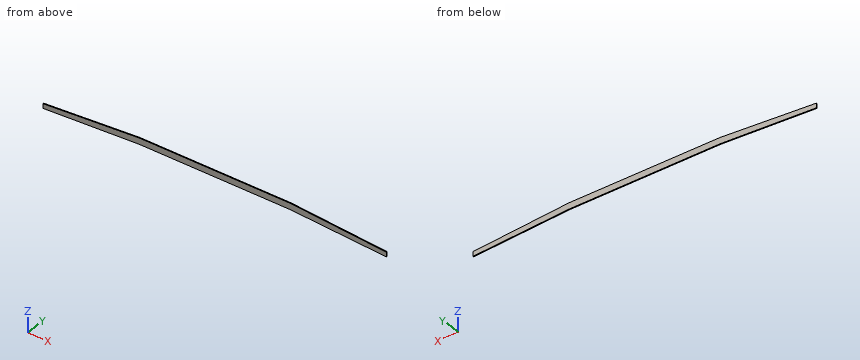
from build123d import *

# Parameters (mm, degrees)
BOSS_EXTRUDE1_DEPTH = 4.3


with BuildPart() as part:
    # Sketch1 → Boss-Extrude1 (new body)
    with BuildSketch(Plane(origin=(0, 0, 0), x_dir=(1, 0, 0), z_dir=(0, 1, 0))):
        Polygon((335.3, -13.5), (762, 17.8), (762, 37.8), (335.3, 13.5), (0, 13.5), (0, -13.5), align=None)
    boss_extrude1 = extrude(amount=BOSS_EXTRUDE1_DEPTH)

    # Mirror1: Boss-Extrude1 across plane
    add(boss_extrude1.mirror(Plane(origin=(0, 4.3, -13.5), x_dir=(0, 0, 1), z_dir=(1, 0, 0))))


solid = part.part
Input: part model. Units: mm. Frame: model coordinates. Round coordinates to 2 decimals unless told otherwise and drop trailing zeros. Write each loop counter-clockwise with the first axis right and the second up, starting at its lowest first coordinate (ties: lowest second). Pieces come first, ordered by that corner, then holes.
1) Cut plane B-B (x = -124). Return the cut outline in (y, z).
2) Contact query for a flat-ended pin moving along its axis: P1, Ø2, axis at x = -19.5, y = 2.5, coming from the -Z side. Output: stop coordinate, or through.
3) Ray query, L1, parallel to Z at x = -237, y = 2.65; L2, parallel to Z at x = -632.5, y = 1.5. Return the intervals inside material, ascending.
4) Cut plane A-A (y = 2.2). Return the cut outline in (x, z), then the cut area to 3 significant figures.
5) Cut plane C-C (z = 0.5). Return the cut outline in (x, y).
Geometry says:
1. outline: (0, -13.5) - (4.3, -13.5) - (4.3, 13.5) - (0, 13.5) - close
2. P1: stops at z = -13.5
3. L1: z = -13.5 to 13.5
3. L2: z = -30.43 to -8.3
4. outline: (-762, -37.8) - (-335.3, -13.5) - (335.3, -13.5) - (762, -37.8) - (762, -17.8) - (335.3, 13.5) - (-335.3, 13.5) - (-762, -17.8) - close
4. area: 38,200 mm2
5. outline: (-512.52, 0) - (512.52, 0) - (512.52, 4.3) - (-512.52, 4.3) - close
